Check sheet for the modelled part. Datum: model origin and axes. Units: mm. Give positions to 0.01 mm unless a question says otherwise; leave off trailing zeros. Loops run counter-clockwise (first coordinate to the right, second up) from the corner with the lowest first, then second, coordinate; pieces in that order, holes last. Notation, with made-up numbers: (1.25, 48.5) - (57.25, 48.5) arc R16 ccw to (57.25, 75.5) - close; hole circle Ø11 at (-5.75, -34). An arc over 180 degrees is marked (long way). Use CSV: the item, a comma, the result in double quotes.
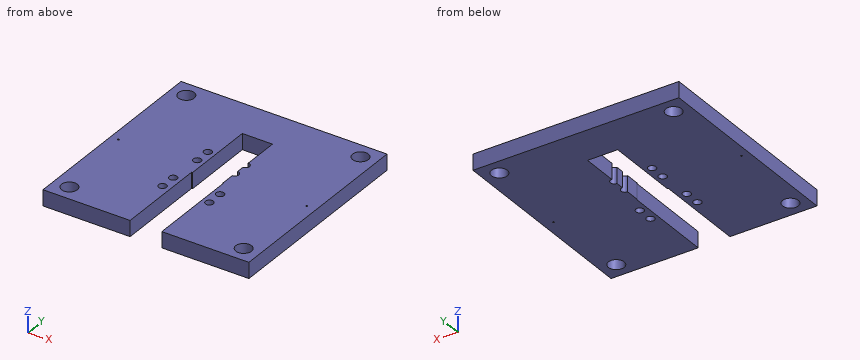
Autodesk Inventor part; units mm, degrees
ref_plane "YZ Plane" through (0, 0, 0) normal (1, 0, 0) x (0, 1, 0)
ref_plane "XZ Plane" through (0, 0, 0) normal (0, 1, 0) x (-1, 0, 0)
ref_plane "XY Plane" through (0, 0, 0) normal (0, 0, 1) x (1, 0, 0)
sketch "Sketch1" plane through (0, 0, 0) normal (0, 0, 1) x (1, 0, 0)
  line L0 (0, 0) -> (130, 0)
  line L1 (130, 0) -> (130, 130)
  line L2 (130, 130) -> (0, 130)
  line L3 (0, 130) -> (0, 0)
  dimension "d0" = 130
  dimension "d1" = 130
extrude "Extrusion1" add sketch "Sketch1" along normal blind 10
sketch "Sketch2" plane through (0, 0, 10) normal (0, 0, 1) x (1, 0, 0)
  line L0 (0, 0) -> (130, 0)
  line L1 (0, 0) -> (10, 0)
  line L2 (10, 0) -> (10, 110)
  line L3 (10, 110) -> (10, 120)
  line L4 (10, 120) -> (120, 120)
  line L5 (120, 120) -> (120, 10)
  line L6 (120, 10) -> (10, 10)
  circle A0 centre (10, 120) radius 5
  circle A1 centre (120, 120) radius 5
  circle A2 centre (10, 10) radius 5
  circle A3 centre (120, 10) radius 5
  dimension "d4" = 10
  dimension "d5" = 110
  dimension "d6" = 10
  dimension "d7" = 110
  dimension "d8" = 110
  dimension "d9" = 110
  dimension "d10" = 10
  dimension "d11" = 10
  dimension "d12" = 10
  dimension "d13" = 10
extrude "Extrusion2" cut sketch "Sketch2" against normal through all contours A2 L2 | L2 L6 A2 | L2 A2 L6 | A3 L5 L6 | L6 L5 A3 | A0 L4 L3 | L3 L4 A0 | A1 L4 L5 | L5 L4 A1
sketch "Sketch3" plane through (0, 0, 10) normal (0, 0, 1) x (1, 0, 0)
  line L0 (0, 0) -> (130, 0)
  line L1 (68.2625, 0) -> (63.2625, 0)
  line L2 (63.2625, 0) -> (63.2625, 5)
  circle A0 centre (63.2625, 5) radius 0.05
  dimension "d16" = 5
  dimension "d17" = 5
  dimension "d18" = 0.1
extrude "Extrusion3" cut sketch "Sketch3" along normal through all both and the other way through all
sketch "Sketch4" plane through (0, 0, 10) normal (0, 0, 1) x (1, 0, 0)
  line L0 (63.5, 131.7625) -> (63.5, 126.7625)
  circle A0 centre (63.5, 126.7625) radius 0.05
  point P0 (0, 0)
  dimension "d21" = 5
  dimension "d22" = 0.1
extrude "Extrusion4" cut sketch "Sketch4" against normal blind 10
sketch "Sketch5" plane through (0, 0, 10) normal (0, 0, 1) x (1, 0, 0)
  line L0 (0, 63.5) -> (5, 63.5)
  line L1 (5, 63.5) -> (123.825, 63.5)
  circle A0 centre (5, 63.5) radius 0.5
  circle A1 centre (123.825, 63.5) radius 0.5
  point P0 (0, 0)
  dimension "d25" = 5
  dimension "d26" = 1
  dimension "d27" = 1
extrude "Extrusion5" cut sketch "Sketch5" against normal through all
sketch "Sketch6" plane through (0, 0, 10) normal (0, 0, 1) x (1, 0, 0)
  point P0 (0, 0)
sketch "Sketch7" plane through (0, 0, 10) normal (0, 0, 1) x (1, 0, 0)
  line L0 (0, 0) -> (55, 0)
  line L1 (0, 0) -> (130, 0)
  line L2 (55, 0) -> (75, 0)
  line L3 (75, 0) -> (130, 0)
  line L4 (55, 0) -> (75, 0)
  line L5 (75, 0) -> (75, 58)
  line L6 (75, 58) -> (55, 58)
  line L7 (55, 58) -> (55, 0)
  dimension "d30" = 55
  dimension "d31" = 20
  dimension "d32" = 55
  dimension "d33" = 20
  dimension "d34" = 58
extrude "Extrusion6" cut sketch "Sketch7" against normal blind 10
sketch "Sketch8" plane through (0, 0, 10) normal (0, 0, 1) x (1, 0, 0)
  line L0 (74.6125, 0) -> (79.6125, 0)
  line L1 (79.6125, 0) -> (79.6125, 38)
  line L2 (79.6125, 38) -> (79.6125, 48)
  line L3 (55, 58) -> (55, 0)
  line L4 (55, 0) -> (50, 0)
  line L5 (0, 0) -> (55, 0)
  line L6 (50, 0) -> (50, 38)
  line L7 (50, 38) -> (50, 48)
  circle A0 centre (79.6125, 48) radius 2.5
  circle A1 centre (79.6125, 38) radius 2.5
  circle A2 centre (50, 48) radius 2.5
  circle A3 centre (50, 38) radius 2.5
  dimension "d37" = 5
  dimension "d38" = 38
  dimension "d39" = 10
  dimension "d40" = 5
  dimension "d41" = 38
  dimension "d42" = 10
  dimension "d43" = 5
  dimension "d44" = 5
  dimension "d45" = 5
  dimension "d46" = 5
extrude "Extrusion7" cut sketch "Sketch8" against normal through all
sketch "Sketch9" plane through (0, 0, 10) normal (0, 0, 1) x (1, 0, 0)
  line L0 (55.5625, 57.15) -> (74.6125, 57.15)
  line L1 (74.6125, 57.15) -> (74.6125, 104.775)
  line L2 (74.6125, 104.775) -> (55.5625, 104.775)
  line L3 (55.5625, 104.775) -> (55.5625, 57.15)
  point P0 (0, 0)
extrude "Extrusion8" cut sketch "Sketch9" against normal blind 10
sketch "Sketch10" plane through (0, 0, 10) normal (0, 0, 1) x (1, 0, 0)
  line L0 (0, 0) -> (55, 0)
  line L1 (55, 0) -> (55, 5)
  line L2 (55, 0) -> (42.8625, 0)
  dimension "d51" = 5
sketch "Sketch11" plane through (0, 0, 10) normal (0, 0, 1) x (1, 0, 0)
  line L0 (55.5625, 0) -> (50.5625, 0)
  line L1 (0, 0) -> (55, 0)
  dimension "d52" = 5
sketch "Sketch12" plane through (0, 0, 10) normal (0, 0, 1) x (1, 0, 0)
  line L0 (75, 58) -> (75, 0)
  line L1 (75, 0) -> (80, 0)
  line L2 (75, 0) -> (130, 0)
  line L3 (80, 0) -> (80, 85.725)
  line L4 (80, 85.725) -> (80, 100.0125)
  line L5 (50.8, 0) -> (50.8, 69.4562)
  line L6 (55, 0) -> (55, 58)
  line L7 (50.8, 69.4562) -> (50.8, 79.4562)
  line L8 (50.8, 79.4562) -> (80, 79.4562)
  circle A0 centre (50.8, 79.4562) radius 2.5
  circle A1 centre (50.8, 69.4562) radius 2.5
  line L9 (50.8, 69.4562) -> (80, 69.4562)
  line L10 (80, 79.4562) -> (82.5, 79.4562)
  line L11 (82.5, 79.4562) -> (77.5, 79.4562)
  line L12 (77.5, 79.4562) -> (77.5, 69.4562)
  circle A2 centre (74.6125, 79.4562) radius 2.5
  circle A3 centre (74.6125, 69.4562) radius 2.5
  point P0 (0, 0)
  dimension "d53" = 5
  dimension "d54" = 10
  dimension "d55" = 5
  dimension "d56" = 5
  dimension "d61" = 2.5
  dimension "d62" = 5
  dimension "d64" = 5
  dimension "d65" = 5
extrude "Extrusion9" cut sketch "Sketch12" against normal blind 10 contours A3 L9 | L9 A3 | A2 L8 | L8 A2 | L9 L7 A1 | A1 L5 L9 | A0 L7 L8 | L8 L7 A0 | L7 L5 A1
properties part number "top STAND PLATE FOR STORSGE SYSTEM"
1. Sectioned sample at D-D, the plane z = 4.75. State how many separate pieces and enclosed holes the cut face has, and give its area (3 significant figures).
Completed:
separate pieces,"1"
enclosed holes,"13"
area,"14,400 mm²"
2. Scan lines: line 1 along X through (y, z) = (48, 8); line 2 along Y through (x, z) = (10.5, 9.5); line 3 along X through (y, z) = (63.5, 5.75) (1 decimal). Record each from-to range of solid material in increasing order.
Completed:
line 1,"x = 0 to 47.5, 52.5 to 55, 75 to 77.11, 82.11 to 130"
line 2,"y = 0 to 5.03, 14.97 to 115.03, 124.97 to 130"
line 3,"x = 0 to 4.5, 5.5 to 55.6, 74.6 to 123.3, 124.3 to 130"
3. Go/stop test with a flat-tipped pin: pin 1 Ø5 at (x, z) = (66.5, 6.5) entering from -Y (3 decimals). Record where the tip stops, or that it passes through.
Completed:
pin 1,"stops at y = 104.775"
4. Sectioned sample at B-B, the plane y = 29. Record the boundary of the cut face in (x, z).
Completed:
outline,"(0, 0) - (55, 0) - (55, 10) - (0, 10) - close; (75, 0) - (130, 0) - (130, 10) - (75, 10) - close"
5. Sectioned sample at C-C, the plane y = 48. Record the boundary of the cut face in (x, z), and give its area (3 significant figures).
Completed:
outline,"(0, 0) - (47.5, 0) - (47.5, 10) - (0, 10) - close; (52.5, 0) - (55, 0) - (55, 10) - (52.5, 10) - close; (75, 0) - (77.11, 0) - (77.11, 10) - (75, 10) - close; (82.11, 0) - (130, 0) - (130, 10) - (82.11, 10) - close"
area,"1,000 mm²"
6. Sectioned sample at A-A, the plane x = 10. Record the boundary of the cut face in (y, z).
Completed:
outline,"(0, 0) - (5, 0) - (5, 10) - (0, 10) - close; (15, 0) - (115, 0) - (115, 10) - (15, 10) - close; (125, 0) - (130, 0) - (130, 10) - (125, 10) - close"
